```python
from build123d import *

# Parameters (mm, degrees)
F4_R      = 53.6942028964
F5_DEPTH  = 10
F6_T      = -1
F11_R     = 7.1329818057
F12_DEPTH = 62.1
F13_R     = 7.1161383354
F14_DEPTH = 79.5
F16_DEPTH = 25


# Not quite as in the source:
# - the program builds the solid bodies; features that only make, move or delete a surface that nothing else refers to are left out


with BuildPart() as f5:
    # F4 (on Top) → F5 (new body)
    with BuildSketch(Plane.XY):
        Circle(F4_R)
    extrude(amount=F5_DEPTH)

    # F6
    f6_openings = [f5.faces().sort_by_distance(p)[0] for p in [
        (0, 0, 10),
    ]]
    offset(amount=F6_T, openings=f6_openings)

    # F11 (on Top) → F12 (cut)
    with BuildSketch(Plane.XY):
        Circle(F11_R)
    extrude(amount=-F12_DEPTH, mode=Mode.SUBTRACT)

    # F13 (on Top) → F14 (cut)
    with BuildSketch(Plane.XY):
        Circle(F13_R)
    extrude(amount=F14_DEPTH, mode=Mode.SUBTRACT)

    # F15 (on face) → F16 (cut)
    with BuildSketch(Plane(origin=(0, 0, 0), x_dir=(1, 0, 0), z_dir=(0, 0, -1))):
        with BuildLine():
            Line((0, 11.3609913542), (12.56390222, 48.5457946048))
            ThreePointArc((12.56390222, 48.5457946048), (-7.6213284004, 49.5626993435), (-26.5685055521, 42.5283473172))
            Line((-26.5685055521, 42.5283473172), (-4.8620371636, 10.2680435901))
            ThreePointArc((-4.8620371636, 10.2680435901), (-2.4916831758, 11.0843871955), (0, 11.3609913542))
        make_face()
        with BuildLine():
            Line((-9.7046168543, 5.9069904572), (-41.6567469595, 27.9152511283))
            ThreePointArc((-41.6567469595, 27.9152511283), (-50.0893104585, 2.3678662526), (-44.1043633563, -23.8610759552))
            Line((-44.1043633563, -23.8610759552), (-11.0760480746, -2.5284943342))
            ThreePointArc((-11.0760480746, -2.5284943342), (-11.2137576056, 1.8231195549), (-9.7046168543, 5.9069904572))
        make_face()
        with BuildLine():
            ThreePointArc((-38.3285737992, -32.3336704276), (-25.4491957444, -43.2074559395), (-9.6943225855, -49.1992471732))
            Line((-9.6943225855, -49.1992471732), (-3.2570755528, -10.8840977298))
            ThreePointArc((-3.2570755528, -10.8840977298), (-5.8587236117, -9.733831835), (-8.0930813532, -7.9733405019))
            Line((-8.0930813532, -7.9733405019), (-38.3285737992, -32.3336704276))
        make_face()
        with BuildLine():
            ThreePointArc((-3.1826565415, -50.0441456131), (17.9564047347, -46.8200100577), (35.8302023129, -35.0819385869))
            Line((35.8302023129, -35.0819385869), (3.9370343752, -10.6570110668))
            ThreePointArc((3.9370343752, -10.6570110668), (1.9997392278, -11.183611562), (0, -11.3609913542))
            Line((0, -11.3609913542), (-3.1826565415, -50.0441456131))
        make_face()
        with BuildLine():
            ThreePointArc((42.8675483184, -26.0176692648), (48.2915604345, -13.5081828387), (50.1452471606, 0))
            ThreePointArc((50.1452471606, 0), (50.1236727364, 1.4707971358), (50.058968028, 2.9403286841))
            Line((50.058968028, 2.9403286841), (11.1284959107, -2.2866358071))
            ThreePointArc((11.1284959107, -2.2866358071), (10.0225700646, -5.3497863368), (8.0930813532, -7.9733405019))
            Line((8.0930813532, -7.9733405019), (42.8675483184, -26.0176692648))
        make_face()
        with BuildLine():
            Line((10.5704846038, 4.1637699011), (47.1017248223, 17.2038754811))
            ThreePointArc((47.1017248223, 17.2038754811), (37.4128970239, 33.3889345305), (22.4298275607, 44.8491766747))
            Line((22.4298275607, 44.8491766747), (5.6516858546, 9.8554843387))
            ThreePointArc((5.6516858546, 9.8554843387), (8.5958482365, 7.4285609403), (10.5704846038, 4.1637699011))
        make_face()
    extrude(amount=-F16_DEPTH, mode=Mode.SUBTRACT)


solid = f5.part
```
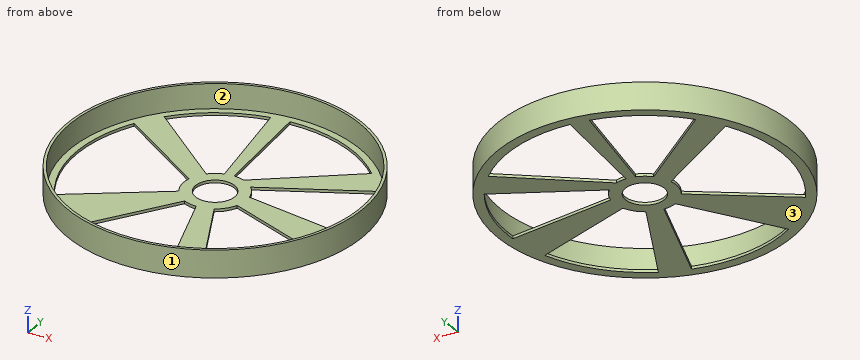
Read the model definition and answer for the solid it produces. Units are mm, in the model's axes. Face numbers are marked on the shaded views. Give positions to 0.01 mm unless a question says otherwise; leave off trailing zeros. Write each loop counter-clockwise with the first axis right and the second up, starting at its lowest first coordinate (ties: lowest second). Pieces come first, ordered by that corner, then holes. Notation, with made-up numbers: (78, 14) - (112, 14) arc R22 ccw to (112, 35) - close; hole circle Ø1 at (88.25, 8). An arc over 180 degrees is marked (long way). Write item = value, one per line. Start each with the question number.
Item 1: Each of these flat-tipped pins is pushed along its axis until it touches: P1, Ø6, axis at y = 30, z = 1.5, coming from the +X side; P2, Ø16.5, axis at x = 0, y = 0, coming from the +Z side; P3, Ø10, axis at x = -26, y = -25.5, coming from the -Z side; P4, Ø6, axis at x = -32, z = 2, coming from the -Y side. Where does it stop, or does it pass through?
Item 2: Find the intervals of material crossed by probe 1 along Z at (x, y) = (-41, -28); probe 2 along X at (y, z) = (-38.5, 6.5); probe 3 along Y at (x, z) = (21, 1.75), in increasing order. Write a range as [from, to].
Item 3: Find section D-D (z = 5.75). Give the vertices of the cut face in (x, y), then the cut area to 3 significant figures.
Item 4: The mould has two halves that part along X. Classify the marked faces 1, 2 and 3: +X half, -X half, draft (parallel to the pull), parting line (faces both ways), or undercut.
Item 5: Find section B-B (y = -24). Give the vertices of the cut face in (x, z).
Item 6: Find section A-A (x = -35.5). Give the vertices of the cut face in (y, z).
Item 7: Find section C-C (x = -22). Give the vertices of the cut face in (y, z), then the cut area to 3 significant figures.
Response:
q1.P1 = 46.41
q1.P2 = 1
q1.P3 = 0
q1.P4 = -45.19
q2.probe_1 = [0, 1]
q2.probe_2 = [-37.43, -35.98], [35.98, 37.43]
q2.probe_3 = [-49.42, -48.33], [48.33, 49.42]
q3.outline = circle Ø107.39 at (0, 0); hole circle Ø105.39 at (0, 0)
q3.area = 334 mm²
q4.face_1 = parting line
q4.face_2 = undercut
q4.face_3 = draft
q5.outline = (-48.03, 0) - (-44.03, 0) - (-44.03, 1) - (-46.91, 1) - (-46.91, 10) - (-48.03, 10) - close; (-35.97, 0) - (-14.1, 0) - (-14.1, 1) - (-35.97, 1) - close; (4.27, 0) - (12.43, 0) - (12.43, 1) - (4.27, 1) - close; (44.03, 0) - (48.03, 0) - (48.03, 10) - (46.91, 10) - (46.91, 1) - (44.03, 1) - close
q6.outline = (-40.28, 0) - (-23.67, 0) - (-23.67, 1) - (-38.94, 1) - (-38.94, 10) - (-40.28, 10) - close; (18.3, 0) - (30.05, 0) - (30.05, 1) - (18.3, 1) - close; (35.42, 0) - (40.28, 0) - (40.28, 10) - (38.94, 10) - (38.94, 1) - (35.42, 1) - close
q7.outline = (-48.98, 0) - (-45.06, 0) - (-45.06, 1) - (-47.88, 1) - (-47.88, 10) - (-48.98, 10) - close; (-35.74, 0) - (-14.38, 0) - (-14.38, 1) - (-35.74, 1) - close; (9.58, 0) - (19.18, 0) - (19.18, 1) - (9.58, 1) - close; (45.06, 0) - (48.98, 0) - (48.98, 10) - (47.88, 10) - (47.88, 1) - (45.06, 1) - close
q7.area = 58.6 mm²
